Autodesk Inventor part; units mm, degrees
ref_plane "Work Plane1" through (0, 0, 11.15) normal (0, 0, 1) x (1, 0, 0)
ref_plane "Work Plane2" through (0, 0, 14.2) normal (0, 0, 1) x (1, 0, 0)
ref_plane "YZ Plane" through (0, 0, 0) normal (1, 0, 0) x (0, 1, 0)
sketch "Sketch1" plane through (0, 0, 0) normal (0, 1, 0) x (-1, 0, 0)
  circle A0 centre (0, 0) radius 7.15
  circle A1 centre (0, 0) radius 11.15
  point P0 (0, 11.15)
  dimension "d1" = 22.3
  dimension "d0" = 14.3
extrude "Small" add sketch "Sketch1" along normal blind 40
sketch "Sketch2" plane through (0, 0, 0) normal (0, -1, 0) x (1, 0, 0)
  circle A0 centre (0, 0) radius 7.15
  circle A1 centre (0, 0) radius 10.2
  circle A2 centre (0, 0) radius 11.15
  circle A3 centre (0, 0) radius 14.2
  point P0 (0, 14.2)
  dimension "d5" = 28.4
  dimension "d4" = 20.4
extrude "Big" add sketch "Sketch2" along normal blind 40 contours A2 | A3
ref_plane "Work Plane1" through (0, 0, 11.15) normal (0, 0, 1) x (1, 0, 0)
ref_plane "Work Plane2" through (0, 0, 14.2) normal (0, 0, 1) x (1, 0, 0)
sketch "Sketch3" plane through (0, 0, 11.15) normal (0, 0, 1) x (1, 0, 0)
  line L0 (11.15, 40) -> (-11.15, 40)
  point P0 (0, 0)
  point P1 (0, 25)
  dimension "d25" = 15
hole "Screw Hole for small" at (0, 25, 11.15) direction (0, 0, -1) diameter 2 end through all
sketch "Sketch4" plane through (0, 0, 14.2) normal (0, 0, 1) x (1, 0, 0)
  line L0 (-14.2, -40) -> (14.2, -40)
  point P0 (0, 0)
  point P1 (0, -25)
  dimension "d24" = 15
hole "Screw Hole for big" at (0, -25, 14.2) direction (0, 0, -1) diameter 2 end through all
fillet "Fillet1 outside" radius 10 2 edges at (-14.2, 0, 0) (11.15, 0, 0)
fillet "Fillet2 Inside" radius 10 1 edges at (-10.2, 0, 0)
fillet "Fillet3" radius 5 2 edges at (0, 0, 7.15) (0, 0, -7.15)
properties part number "hollowCylinderTest_3DPrint"
Input: part model. Units: mm. Frame: model coordinates. A direction names the side the tool comes from. Round coordinates to 2 decimals unless told otherwise and drop trailing zeros. Write each loop counter-clockwise with the first axis right and the second up, starting at its lowest first coordinate (ties: lowest second). Pieces come first, ordered by that corner, then holes.
1) Contact query for flat-ended pins moving along their axis: P1, Ø10, axis at y = -19.5, z = -7.5, coming from the +X side; P2, Ø1.6, axis at x = 0, y = 25, coming from the +Z side; P3, Ø2.5, axis at x = 0, y = 25, coming from the +Z side; P4, Ø4, axis at y = 27.5, z = 3, coming from the -X side. Output: stop coordinate, or through.
2) Reachability of faces 4 (the cylindrical face through (0, 24, -9)), 5 (the cylindrical face through (-10.635, 21.457, -3.349)) from +Z, -Z, +X, -X, +Y, -Y: full face, straight path, thin tool, end or side. Return the list, or none.
3) Cut plane B-B (y = -22). Return the cut outline in (x, z).
4) Cut plane C-C (x = 0). Count the separate pieces of the cut face and the enclosed holes in it, then the cut area to 3 significant figures.
5) Draft query along Y for faces 1 (the cylindrical face through (4.707, -23.365, 9.049)), 2 (the cylindrical face through (0, -26, -12)), 3 (the flat face through (-10, -40, 3)). Return one class per face: pulls with the +Y half, pulls with the -Y half, needs draft (parallel to the pull), parting line crosses it, or undercut.
6) Ray query, L1, parallel to Z at x = 0, y = -23; L2, parallel to Z at x = -5, y = -34; L3, parallel to X at y = -25, z = -13.1. Return the intervals inside material, ascending.
Geometry says:
1. P1: stops at x = 13.98
1. P2: passes through
1. P3: stops at z = 11.15
1. P4: stops at x = -11.11
2. face 4: +Z, -Z
2. face 5: +Y
3. outline: circle Ø28.4 at (0, 0); hole circle Ø20.4 at (0, 0)
4. separate pieces: 6
4. enclosed holes: 0
4. area: 609 mm2
5. face 1: needs draft
5. face 2: undercut
5. face 3: pulls with the -Y half
6. L1: z = -14.2 to -10.2, 10.2 to 14.2
6. L2: z = -13.29 to -8.89, 8.89 to 13.29
6. L3: x = -5.48 to -1, 1 to 5.48
